```python
from build123d import *

# Parameters (mm, degrees)
F1_DEPTH = 5.08


with BuildPart() as f1:
    # F0 (on Top) → F1 (new body)
    with BuildSketch(Plane.XY):
        with BuildLine():
            Line((-17.206924, 4.943109), (-47.369424, 4.943109))
            Line((-47.369424, 4.943109), (-47.369424, 0.180609))
            Line((-47.369424, 0.180609), (-29.087516, -4.581891))
            Line((-29.087516, -4.581891), (11.064883, -4.581891))
            ThreePointArc((11.064883, -4.581891), (15.564746, -0.082027), (20.064609, -4.581891))
            Line((20.064609, -4.581891), (37.086151, -4.581891))
            Line((37.086151, -4.581891), (37.086151, 4.943109))
            Line((37.086151, 4.943109), (19.306151, 4.943109))
            Line((19.306151, 4.943109), (12.955576, 4.943109))
            Line((12.955576, 4.943109), (-17.206924, 4.943109))
        make_face()
    extrude(amount=F1_DEPTH)


solid = f1.part
```
Part model, mm, in its own coordinate system. Round coordinates to 2 decimals unless told otherwise and drop trailing zeros. Loops run counter-clockwise (first coordinate to the right, second up) from the corner with the lowest first, then second, coordinate; pieces in that order, holes last.
Item 1: Mould opens along X. For faces 1 (the face through (28, -4.582, 3)), 2 (the face through (37.086, 0, 3)), 3 (the face through (15.466, -0.083, 2.504)), 4 (the face through (-38.356, -2.167, 2.504)) say: +X half, -X half, draft (parallel to the pull), parting line (faces both ways), or undercut.
Item 2: Cut at A-A, the plane z = 2.95. Give the cut face in (x, y), then the cut area to 3 significant figures.
Item 3: Cut at B-B, the plane y = -1. Give the cut face in (x, z).
Item 4: Cut at D-D, the plane x = 12.5. Give the cut face in (y, z), then the cut area to 3 significant figures.
Item 5: Cut at C-C, the plane x = -41. Give the cut face in (y, z), then the cut area to 3 significant figures.
Item 6: Drill centre line: line 1 (Y direction, x = 19.5, z = 1.1). Where is it in solid material? Low to high.
A:
1. face 1: draft
1. face 2: +X half
1. face 3: undercut
1. face 4: -X half
2. outline: (-47.37, 0.18) - (-29.09, -4.58) - (11.06, -4.58) arc R4.5 cw to (20.06, -4.58) - (37.09, -4.58) - (37.09, 4.94) - (-47.37, 4.94) - close
2. area: 729 mm2
3. outline: (-42.84, 0) - (12.84, 0) - (12.84, 5.08) - (-42.84, 5.08) - close; (18.29, 0) - (37.09, 0) - (37.09, 5.08) - (18.29, 5.08) - close
4. outline: (-1.29, 0) - (4.94, 0) - (4.94, 5.08) - (-1.29, 5.08) - close
4. area: 31.6 mm2
5. outline: (-1.48, 0) - (4.94, 0) - (4.94, 5.08) - (-1.48, 5.08) - close
5. area: 32.6 mm2
6. line 1: y = -2.4 to 4.94
